```python
from build123d import *

# Parameters (mm, degrees)
SKETCH2_W           = 64
SKETCH2_H           = 64
BOSS_EXTRUDE1_DEPTH = 1
SKETCH3_W           = 20
SKETCH3_H           = 43
BOSS_EXTRUDE2_DEPTH = 12
BOSS_EXTRUDE3_DEPTH = 10


with BuildPart() as part:
    # Sketch2 → Boss-Extrude1 (new body)
    with BuildSketch(Plane.XY):
        with Locations((32, 32)):
            Rectangle(SKETCH2_W, SKETCH2_H)
    extrude(amount=BOSS_EXTRUDE1_DEPTH)

    # Sketch3 → Boss-Extrude2 (add)
    with BuildSketch(Plane.XY):
        with Locations((8.5, 32)):
            Rectangle(SKETCH3_W, SKETCH3_H)
        with Locations((55.5, 32)):
            Rectangle(SKETCH3_W, SKETCH3_H)
    extrude(amount=-BOSS_EXTRUDE2_DEPTH)

    # Sketch5 → Boss-Extrude3 (add)
    with BuildSketch(Plane(origin=(27, 0, 0), x_dir=(0, 0, -1), z_dir=(1, 0, 0))):
        Polygon((11.654534966, 3.002134122), (4.730028144, 2), (0, 2), (0, 12), (4.730028144, 12), (11.654534966, 8.002134122), align=None)
        Polygon((0, 62), (0, 52), (4.730028144, 52), (11.654534966, 55.997865878), (11.654534966, 60.997865878), (4.730028144, 62), align=None)
    extrude(amount=BOSS_EXTRUDE3_DEPTH)


solid = part.part
```
For this review, take the finished solid that the model builds, in its own axes (mm). A direction names the side the tool comes from. Give positions to 0.01 mm unless a question says otherwise; leave off trailing zeros. Order: outer loops, then holes, each group sorted by start corner. A loop starts at its lowest first (then second) coordinate and runs counter-clockwise, first axis right, second up.
1) Take a section at B-B (y = 7). Give the boundary of the cut face in (x, z).
2) For faces 5 (the face through (-1, 32, 0)), 6 (the face through (65, 32, 0)), 7 (the face through (32, 12, -2)), list the 3-axis set-ups (+Z, -Z, +X, -X, +Y, -Y) from which the entire face can be reached by the end or side of a thin tool; tool diameter is ignored.
3) Take a section at C-C (x = 59). Give the boundary of the cut face in (y, z), then the cut area to 3 significant figures.
4) Take a section at D-D (z = -10.25). Give the boundary of the cut face in (x, y), then the cut area to 3 significant figures.
5) Take a section at A-A (z = -1). Give the boundary of the cut face in (x, y).
6) The part is to be moulded in two halves that separate along Y. For faces 1 (the face through (32, 52, -2)), 2 (the face through (37, 57, -6)), 3 (the face through (8, 53.5, -6)), 4 (the face through (32, 2, -2)), say which applies: released by +Y, released by -Y, zero draft, split by the parting line, or undercut.
7) Insertion check: pin 1 (4 mm diameter, centred on x = 30, z = -3.5, fed in from +Y); pin 2 (1.2 mm diameter, centred on x = -1, y = 28.5, fed in from +Z); pin 3 (5 mm diameter, centred on y = 59, z = -4.5, fed in from +X). Each pin has a flat end and moves straight along its axis. Give the tip position at first contact, or say it passes through.
8) Wall thickness on line 1 (X direction, y = 53, z = -2.25); line 2 (X direction, y = 23, z = -10.25); line 3 (X direction, y = 9.5, z = -8): over which ranges is each line inside the solid? List them lowest first.
Derived:
1. outline: (0, 0) - (27, 0) - (27, -11.65) - (37, -11.65) - (37, 0) - (64, 0) - (64, 1) - (0, 1) - close
2. face 5: +Z, -X, +Y, -Y
2. face 6: +Z, +X, +Y, -Y
2. face 7: -Z
3. outline: (0, 0) - (10.5, 0) - (10.5, -12) - (53.5, -12) - (53.5, 0) - (64, 0) - (64, 1) - (0, 1) - close
3. area: 580 mm2
4. outline: (-1.5, 10.5) - (18.5, 10.5) - (18.5, 53.5) - (-1.5, 53.5) - close; (27, 2.8) - (37, 2.8) - (37, 8.81) - (27, 8.81) - close; (27, 55.19) - (37, 55.19) - (37, 61.2) - (27, 61.2) - close; (45.5, 10.5) - (65.5, 10.5) - (65.5, 53.5) - (45.5, 53.5) - close
4. area: 1,840 mm2
5. outline: (-1.5, 10.5) - (18.5, 10.5) - (18.5, 53.5) - (-1.5, 53.5) - close; (27, 2) - (37, 2) - (37, 12) - (27, 12) - close; (27, 52) - (37, 52) - (37, 62) - (27, 62) - close; (45.5, 10.5) - (65.5, 10.5) - (65.5, 53.5) - (45.5, 53.5) - close
6. face 1: undercut
6. face 2: zero draft
6. face 3: released by +Y
6. face 4: released by -Y
7. pin 1: stops at y = 62
7. pin 2: stops at z = 0
7. pin 3: stops at x = 37
8. line 1: x = -1.5 to 18.5, 27 to 37, 45.5 to 65.5
8. line 2: x = -1.5 to 18.5, 45.5 to 65.5
8. line 3: x = 27 to 37
